Verification items for the finished model (mm, model axes). A direction names the side the tool comes from. Coordinates: 2 decimals unless noted, no trailing zeros. Loops run counter-clockwise (first coordinate to the right, second up) from the corner with the lowest first, then second, coordinate; pieces in that order, holes last. Notation, with made-up numbers: (83.25, 56) -> (135.25, 56) arc R12 ccw to (135.25, 79) -> close; hole circle Ø6 at (82, 86.5). An arc over 180 degrees is marked (long way). Answer as a JSON object with one key per item and string values. Group by question number.
Q1. Cross-section at C-C on x = 79.5. Record the boundary of the cut face in (y, z) (3 decimals).
Q2. Cross-section at A-A on x = 144.78. Record the boundary of the cut face in (y, z) (3 decimals).
Q3. Scan lines: L1, parallel to Y at x = 33.02, z = -1.15; L2, parallel to Y at x = 88.9, z = -2.2; L3, parallel to X at y = 75, z = -0.4. Record each from-to range of solid material in increasing order.
Q4. Cross-section at D-D on z = -2.65. Give the number of separate pieces and of enclosed holes in the cut face, and give its area (3 significant figures).
Q5. Gauge pin test, flat ends, axial feed: pin 1 Ø1 at (y, z) = (59.5, -1) entering from -X; pin 2 Ø1.5 at (y, z) = (23.5, -2) entering from +X. Record the tip position at first contact, or that the pin passes through.
Q6. Cross-section at B-B on y = 16.51. Record the boundary of the cut face in (x, z) (3 decimals).
Q7. Set-up check for faces 1 (the flat face through (3.048, 53, -2)), 2 (the cylindrical face through (7.64, 94.36, -1.57)), 3 (the flat face through (174.752, 53, -2)), 4 (the flat face through (90, 101.6, -2)), 5 (the cylindrical face through (54.53, 46.99, -1.57)): record each of +Z, -Z, +X, -X, +Y, -Y from which the full face is reachable in a straight line by a thin tool's end or side.
Autodesk Inventor part; units mm, degrees
ref_plane "Work Plane1" through (25.4, 50.8, 0) normal (0, 1, 0) x (1, 0, 0)
ref_plane "Work Plane2" through (174.752, 25.4, 0) normal (1, 0, 0) x (0, 0, -1)
ref_plane "YZ Plane" through (0, 0, 0) normal (1, 0, 0) x (0, 1, 0)
sketch "Sketch3" plane through (0, 0, 0) normal (0, 0, 1) x (1, 0, 0)
  line L0 (0, 0) -> (177.8, 0)
  line L1 (177.8, 0) -> (177.8, 101.6)
  line L2 (177.8, 101.6) -> (0, 101.6)
  line L3 (0, 101.6) -> (0, 0)
  arc A0 (25.4, 101.6) -> (0, 76.2) centre (25.4, 76.2) ccw
  arc A1 (177.8, 76.2) -> (152.4, 101.6) centre (152.4, 76.2) ccw
  arc A2 (152.4, 0) -> (177.8, 25.4) centre (152.4, 25.4) ccw
  arc A3 (0, 25.4) -> (25.4, 0) centre (25.4, 25.4) ccw
  circle A4 centre (88.9, 50.8) radius 6.35
  arc A5 (88.9, 85.09) -> (54.61, 50.8) centre (88.9, 50.8) ccw construction
  arc A6 (88.9, 88.9) -> (50.8, 50.8) centre (88.9, 50.8) ccw
  arc A7 (88.9, 81.28) -> (58.42, 50.8) centre (88.9, 50.8) ccw
  arc A8 (88.9, 81.28) -> (88.9, 88.9) centre (88.9, 85.09) ccw
  arc A9 (50.8, 50.8) -> (58.42, 50.8) centre (54.61, 50.8) ccw
  line L4 (88.9, 50.8) -> (54.61, 50.8) construction
  line L5 (88.9, 50.8) -> (88.9, 85.09) construction
  arc A10 (88.9, 20.32) -> (119.38, 50.8) centre (88.9, 50.8) ccw
  line L6 (88.9, 50.8) -> (123.19, 50.8) construction
  arc A11 (88.9, 16.51) -> (123.19, 50.8) centre (88.9, 50.8) ccw construction
  arc A12 (127, 50.8) -> (119.38, 50.8) centre (123.19, 50.8) ccw
  arc A13 (88.9, 12.7) -> (127, 50.8) centre (88.9, 50.8) ccw
  arc A14 (88.9, 20.32) -> (88.9, 12.7) centre (88.9, 16.51) ccw
  dimension "d20" = 177.8
  dimension "d21" = 101.6
  dimension "d22" = 50.8
  dimension "d23" = 50.8
  dimension "d24" = 50.8
  dimension "d25" = 50.8
  dimension "d26" = 12.7
  dimension "d27" = 50.8
  dimension "d28" = 88.9
  dimension "d29" = 34.29
  dimension "d30" = 90
  dimension "d31" = 7.62
  dimension "d34" = 360
extrude "Extrusion3" add sketch "Sketch3" against normal blind 3.175 contours A3 L3 A0 L2 A1 L1 A2 L0
ref_plane "Work Plane1" through (25.4, 50.8, 0) normal (0, 1, 0) x (1, 0, 0)
sketch "Sketch4" plane through (0, 0, 0) normal (0, 0, 1) x (1, 0, 0)
  line L0 (0, 76.2) -> (0, 25.4)
  line L1 (0, 50.8) -> (177.8, 50.8)
  line L2 (177.8, 76.2) -> (177.8, 25.4)
  line L3 (152.4, 101.6) -> (25.4, 101.6)
  line L4 (88.9, 101.6) -> (88.9, 0)
  circle A0 centre (12.7, 71.882) radius 6.35
  circle A1 centre (33.02, 71.882) radius 6.35
  line L5 (0, 25.4) -> (0, 76.2)
  circle A2 centre (12.7, 29.718) radius 6.35
  circle A3 centre (33.02, 29.718) radius 6.35
  circle A4 centre (165.1, 71.882) radius 6.35
  circle A5 centre (144.78, 71.882) radius 6.35
  circle A6 centre (165.1, 29.718) radius 6.35
  circle A7 centre (144.78, 29.718) radius 6.35
  point P0 (0, 0)
  dimension "d39" = 12.7
  dimension "d40" = 12.7
  dimension "d41" = 20.32
  dimension "d42" = 12.7
  dimension "d43" = 21.082
extrude "Extrusion4" cut sketch "Sketch4" against normal blind 25.4
sketch "Sketch5" plane through (177.8, 25.4, 0) normal (1, 0, 0) x (0, 0, -1)
  line L0 (3.175, 50.8) -> (3.175, 76.2)
  line L1 (0, -25.4) -> (3.175, -25.4)
  line L2 (3.175, -25.4) -> (3.175, 50.8)
  line L3 (3.175, 50.8) -> (0, 50.8)
  line L4 (0, 50.8) -> (0, -25.4)
extrude "Extrusion5" cut sketch "Sketch5" against normal blind 3.048
sketch "Sketch6" plane through (0, 25.4, 0) normal (-1, 0, 0) x (0, 0, 1)
  line L0 (0, 50.8) -> (-3.175, 50.8)
  line L1 (-3.175, 50.8) -> (0, 50.8)
  line L2 (0, 50.8) -> (0, -25.4)
  line L3 (0, -25.4) -> (-3.175, -25.4)
  line L4 (-3.175, -25.4) -> (-3.175, 50.8)
extrude "Extrusion6" cut sketch "Sketch6" against normal blind 3.048
sketch "Sketch7" plane through (25.4, 0, 0) normal (0, -1, 0) x (1, 0, 0)
  line L0 (-22.352, -3.175) -> (-22.352, 0)
  line L1 (127, -3.175) -> (152.4, -3.175)
  line L2 (-22.352, 0) -> (149.352, 0)
  line L3 (149.352, 0) -> (149.352, -3.175)
  line L4 (149.352, -3.175) -> (-22.352, -3.175)
  line L5 (-22.352, -3.175) -> (-22.352, 0)
  point P0 (-25.4, 0)
  point P1 (149.352, -1.5875)
  dimension "d50" = 171.704
extrude "Extrusion7" cut sketch "Sketch7" against normal blind 3.048
sketch "Sketch8" plane through (0, 0, 0) normal (0, 0, 1) x (1, 0, 0)
  arc A0 (3.048, 28.448) -> (28.448, 3.048) centre (28.448, 28.448) ccw
  arc A1 (149.352, 3.048) -> (174.752, 28.448) centre (149.352, 28.448) ccw
  line L0 (174.752, 13.3357) -> (174.752, 76.2)
  line L1 (13.3357, 3.048) -> (164.4643, 3.048)
  line L2 (3.048, 76.2) -> (3.048, 13.3357)
  line L3 (3.048, 28.448) -> (3.048, 3.048)
  line L4 (3.048, 3.048) -> (28.448, 3.048)
  line L5 (174.752, 28.448) -> (174.752, 3.048)
  line L6 (174.752, 3.048) -> (149.352, 3.048)
  point P0 (0, 0)
  point P1 (3.048, 13.3357)
  dimension "d53" = 50.8
  dimension "d54" = 50.8
extrude "Extrusion8" cut sketch "Sketch8" against normal through all
ref_plane "Work Plane2" through (174.752, 25.4, 0) normal (1, 0, 0) x (0, 0, -1)
properties part number "Plate"
Computed values:
{
 "1": {"outline": "(3.048, -3.175) -> (79.794, -3.175) -> (79.794, 0) -> (3.048, 0) -> close; (87.722, -3.175) -> (101.6, -3.175) -> (101.6, 0) -> (87.722, 0) -> close"},
 "2": {"outline": "(3.048, -3.175) -> (23.368, -3.175) -> (23.368, 0) -> (3.048, 0) -> close; (36.068, -3.175) -> (65.532, -3.175) -> (65.532, 0) -> (36.068, 0) -> close; (78.232, -3.175) -> (101.6, -3.175) -> (101.6, 0) -> (78.232, 0) -> close"},
 "3": {"L1": "y = 3.05 to 23.37, 36.07 to 65.53, 78.23 to 101.6", "L2": "y = 3.05 to 12.7, 20.32 to 44.45, 57.15 to 81.28, 88.9 to 101.6", "L3": "x = 3.05 to 7.17, 18.23 to 27.49, 38.55 to 59.47, 70.37 to 139.25, 150.31 to 159.57, 170.63 to 174.75"},
 "4": {"separate pieces": "1", "enclosed holes": "11", "area": "14,500 mm²"},
 "5": {"pin 1": "stops at x = 3.05", "pin 2": "stops at x = 174.4"},
 "6": {"outline": "(6.028, -3.175) -> (85.09, -3.175) -> (85.09, 0) -> (6.028, 0) -> close; (105.507, -3.175) -> (171.772, -3.175) -> (171.772, 0) -> (105.507, 0) -> close"},
 "7": {"face 1": "+Z, -Z, -X, -Y", "face 2": "+Z, -Z, -X, +Y", "face 3": "+Z, -Z, +X, -Y", "face 4": "+Z, -Z, +X, -X, +Y", "face 5": "+Z, -Z"}
}
